```python
from build123d import *

# Parameters (mm, degrees)
P_IDAT_VYSUNUT_M1_DEPTH = 5


with BuildPart() as part:
    # Skica1 → Přidat vysunutím1 (new body)
    with BuildSketch(Plane.XY):
        with BuildLine():
            Line((17.662287798, -11.471059771), (11.386287798, -11.471059771))
            Line((11.386287798, -11.471059771), (9.037287798, -11.471059771))
            ThreePointArc((9.037287798, -11.471059771), (8.678077553, -11.322270016), (8.529287798, -10.963059771))
            Line((8.529287798, -10.963059771), (8.529287798, -10.237140432))
            ThreePointArc((8.529287798, -10.237140432), (8.567956995, -10.042737249), (8.678077553, -9.877930187))
            Line((8.678077553, -9.877930187), (11.781158214, -6.774849526))
            ThreePointArc((11.781158214, -6.774849526), (11.945965275, -6.664728968), (12.140368459, -6.626059771))
            Line((12.140368459, -6.626059771), (16.908207136, -6.626059771))
            ThreePointArc((16.908207136, -6.626059771), (17.10261032, -6.664728968), (17.267417381, -6.774849526))
            Line((17.267417381, -6.774849526), (20.370498042, -9.877930187))
            ThreePointArc((20.370498042, -9.877930187), (20.4806186, -10.042737249), (20.519287798, -10.237140432))
            Line((20.519287798, -10.237140432), (20.519287798, -10.963059771))
            ThreePointArc((20.519287798, -10.963059771), (20.370498042, -11.322270016), (20.011287798, -11.471059771))
            Line((20.011287798, -11.471059771), (17.662287798, -11.471059771))
        make_face()
    extrude(amount=-P_IDAT_VYSUNUT_M1_DEPTH)


solid = part.part
```
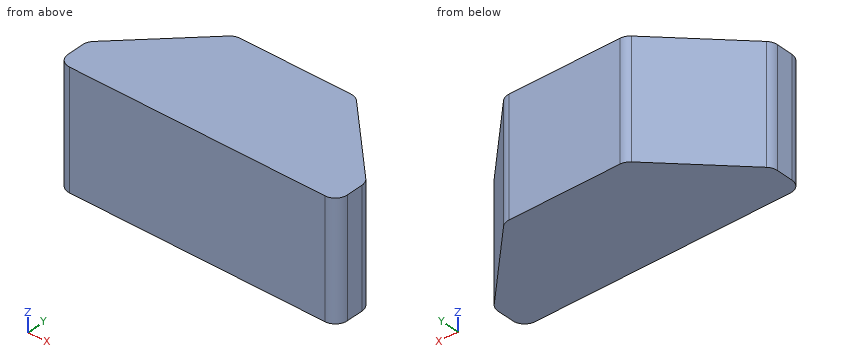
Geometry check sheet. Reference: the model listing, model coordinates, mm. Coordinates: 2 decimals unless noted, no trailing zeros. Order: outer loops, then holes, each group sorted by start corner. A loop starts at its lowest first (then second) coordinate and runs counter-clockwise, first axis right, second up. Notation, with made-up numbers: (38.25, -24.5) - (56.25, -24.5) arc R27 ccw to (56.25, -1.5) - close; hole circle Ø8 at (65, 67). An arc over 180 degrees is marked (long way). Answer in a Markdown table with one row per item. Add a question column.
1. Section check C-C (x = 11.25). Enter the section's corners in (y, z).
2. Material ranges on L1, parallel to X at y = -8.95, z = -0.9; L2, parallel to X at y = -9.55, z = -1; L3, parallel to Y at x = 9.5, z = -0.4, recorded low to high. Write a range as [from, to].
3. Section check A-A (z = -3.8). Enter the section's corners in (x, y), plus the area to 3 significant figures.
4. Section check B-B (y = -8.2). Enter the section's corners in (x, z), plus the area to 3 significant figures.
5. Gauge pin test, flat end, axial feed: pin 1 Ø2 at (x, z) = (10.5, -3.5) entering from +Y. Record the tip position at first contact, or that the pin passes through.
Data:
| question | item | result |
|---|---|---|
| 1 | outline | (-11.47, -5) - (-7.31, -5) - (-7.31, 0) - (-11.47, 0) - close |
| 2 | L1 | x = [9.61, 19.44] |
| 2 | L2 | x = [9.01, 20.04] |
| 2 | L3 | y = [-11.47, -9.06] |
| 3 | outline | (8.53, -10.96) arc R0.51 ccw to (9.04, -11.47) - (20.01, -11.47) arc R0.51 ccw to (20.52, -10.96) - (20.52, -10.24) arc R0.51 ccw to (20.37, -9.88) - (17.27, -6.77) arc R0.51 ccw to (16.91, -6.63) - (12.14, -6.63) arc R0.51 ccw to (11.78, -6.77) - (8.68, -9.88) arc R0.51 ccw to (8.53, -10.24) - close |
| 3 | area | 46.4 mm² |
| 4 | outline | (10.36, -5) - (18.69, -5) - (18.69, 0) - (10.36, 0) - close |
| 4 | area | 41.7 mm² |
| 5 | pin 1 | stops at y = -7.06 |
